from build123d import *

# Parameters (mm, degrees)
SKETCH1_W           = 10.16
SKETCH1_H           = 19.05
BOSS_EXTRUDE1_DEPTH = 6.35
SKETCH2_W           = 6.35
SKETCH2_H           = 15.24
CUT_EXTRUDE1_DEPTH  = 11.16
SKETCH3_W           = 5.08
SKETCH3_H           = 1.27
CUT_EXTRUDE2_DEPTH  = 20.05
SKETCH4_W           = 0.762
SKETCH4_H           = 7.62
CUT_EXTRUDE3_DEPTH  = 11.16
SKETCH5_R           = 2.2098
CUT_EXTRUDE4_DEPTH  = 13.7


with BuildPart() as part:
    # Sketch1 → Boss-Extrude1 (new body, symmetric)
    with BuildSketch(Plane.XY):
        Rectangle(SKETCH1_W, SKETCH1_H)
    extrude(amount=BOSS_EXTRUDE1_DEPTH, both=True)

    # Sketch2 → Cut-Extrude1 (cut, through all)
    with BuildSketch(Plane(origin=(5.08, 0, 0), x_dir=(0, 0, -1), z_dir=(1, 0, 0))):
        with Locations((3.175, -1.905)):
            Rectangle(SKETCH2_W, SKETCH2_H)
    extrude(amount=-CUT_EXTRUDE1_DEPTH, mode=Mode.SUBTRACT)

    # Sketch3 → Cut-Extrude2 (cut, through all)
    with BuildSketch(Plane(origin=(0, 9.525, 0), x_dir=(1, 0, 0), z_dir=(0, 1, 0))):
        with Locations((0, 5.715)):
            Rectangle(SKETCH3_W, SKETCH3_H)
    extrude(amount=-CUT_EXTRUDE2_DEPTH, mode=Mode.SUBTRACT)

    # Sketch4 → Cut-Extrude3 (cut, through all)
    with BuildSketch(Plane(origin=(5.08, 0, 0), x_dir=(0, 0, -1), z_dir=(1, 0, 0))):
        with Locations((-0.381, -3.175)):
            Rectangle(SKETCH4_W, SKETCH4_H)
    extrude(amount=-CUT_EXTRUDE3_DEPTH, mode=Mode.SUBTRACT)

    # Sketch5 → Cut-Extrude4 (cut, through all)
    with BuildSketch(Plane.XY.offset(6.35)):
        with Locations((1.27, 1.905)):
            Circle(SKETCH5_R)
    extrude(amount=-CUT_EXTRUDE4_DEPTH, mode=Mode.SUBTRACT)


solid = part.part
Verification items for the finished model (mm, model axes). A direction names the side the tool comes from. Coordinates: 2 decimals unless noted, no trailing zeros. Write each loop counter-clockwise with the first axis right and the second up, starting at its lowest first coordinate (ties: lowest second). Pieces come first, ordered by that corner, then holes. Notation, with made-up numbers: M -0.5,24 L 26.5,24 A17 ccw 26.5,43 Z; hole C -34,70.5 d10. An arc over 180 degrees is marked long. Use a Markdown table: item, result.
Q1. Sectioned sample at B-B, the plane y = 2.5. Record the boundary of the cut face in (x, z), plus the area to 3 significant figures.
Reply:
| item | result |
|---|---|
| outline | M -5.08,0 L -0.86,0 L -0.86,6.35 L -5.08,6.35 Z; M 3.4,0 L 5.08,0 L 5.08,6.35 L 3.4,6.35 Z |
| area | 37.5 mm² |
Q2. Set-up check for faces 4 (the face through (0, 9.525, 0)), 5 (the face through (-2.54, 8, -6)), 6 (the face through (0, 5.715, -3)): record each of +Z, -Z, +X, -X, +Y, -Y from which the full face is reachable in a straight line by a thin tool's end or side.
Reply:
| item | result |
|---|---|
| face 4 | +Z, -Z, +X, -X, +Y |
| face 5 | -Z, +Y, -Y |
| face 6 | -Z, +X, -X, -Y |
Q3. Sectioned sample at A-A, the plane x = 1.27. Record the boundary of the cut face in (y, z) (3 decimals).
Reply:
| item | result |
|---|---|
| outline | M -9.525,0 L -6.985,0 L -6.985,0.762 L -0.305,0.762 L -0.305,6.35 L -9.525,6.35 Z; M 4.115,0 L 5.715,0 L 5.715,-5.08 L 9.525,-5.08 L 9.525,6.35 L 4.115,6.35 Z |
Q4. Draft check along X on faces 1 (the face through (2.54, 8, -6)), 2 (the face through (0, -3, 0.762)), 3 (the face through (5.08, 2, 2)). Enter one of: +X half, -X half, draft (parallel to the pull), parting line (faces both ways), or undercut.
Reply:
| item | result |
|---|---|
| face 1 | undercut |
| face 2 | draft |
| face 3 | +X half |
Q5. Sectioned sample at C-C, the plane y = 6.5. Record the boundary of the cut face in (x, z), plus the area to 3 significant figures.
Reply:
| item | result |
|---|---|
| outline | M -5.08,-6.35 L -2.54,-6.35 L -2.54,-5.08 L 2.54,-5.08 L 2.54,-6.35 L 5.08,-6.35 L 5.08,6.35 L -5.08,6.35 Z |
| area | 123 mm² |
Q6. Go/stop test with flat-tipped pins: P1, Ø1.5, axis at x = 0, y = 4.5, coming from the -Z side; P2, Ø4, axis at x = 0.5, y = 8.5, coming from the -Z side; P3, Ø4, axis at x = 2, y = -4, coming from the -Z side. Record where each tip stops, or that it passes through.
Reply:
| item | result |
|---|---|
| P1 | stops at z = 0 |
| P2 | stops at z = -5.08 |
| P3 | stops at z = 0.76 |
Q7. Sectioned sample at D-D, the plane z = -4. Record the boundary of the cut face in (x, y) (3 decimals), plus the area to 3 significant figures.
Reply:
| item | result |
|---|---|
| outline | M -5.08,5.715 L 5.08,5.715 L 5.08,9.525 L -5.08,9.525 Z |
| area | 38.7 mm² |
Q8. Thickness scan on line 1 (Y direction, x = 1.27, z = 3.75) (3 decimals); line 2 (X direction, y = 2, z = 3.25); line 3 (Y direction, x = -1.5, z = 0.5) (3 decimals). Record the ranges inside material, lowest first.
Reply:
| item | result |
|---|---|
| line 1 | y = -9.525 to -0.305, 4.115 to 9.525 |
| line 2 | x = -5.08 to -0.94, 3.48 to 5.08 |
| line 3 | y = -9.525 to -6.985, 0.635 to 9.525 |
